Build history of the part. All positions in model axes, mm. Face numbers are marked on the shaded views. A direction names the side the tool comes from. Give positions to 0.01 mm unless a question says otherwise; leave off trailing zeros. Loops run counter-clockwise (first coordinate to the right, second up) from the corner with the lowest first, then second, coordinate; pieces in that order, holes last.
1) Wall check: line 1 (Y direction, x = 33.25, z = 46); line 2 (Y direction, x = 32.25, z = 42); line 3 (Y direction, x = 42.25, z = 41). Give the ranges that are in metal, low to high.
2) Band-saw the part on B-B on x = 37. State how many separate pieces and enclosed holes the cut face has, then the cut area to 3 significant figures.
3) Flat gauge pins, fed straight in: P1, Ø4.5, axis at y = 71.37, z = 65, coming from the -X side; P2, Ø5, axis at x = 43, z = 27.5, coming from the -Y side. Where does each tip first touch, or does it go through?
4) Two-plate mould, pull along Z, no slides. Class the marked faces 1, 2, 3 and 4: +Z half, -Z half, draft (parallel to the pull), parting line (faces both ways), or undercut.
5) Band-saw the part on A-A on z = 27. List the corners of the cut face in (x, y).
6) 3-axis set-ups, long thin cutter, end or side, ignore diameter. For the marked faces 5 and 6: which of +Z, -Z, +X, -X, +Y, -Y reach the whole face in a straight line?
```python
from build123d import *

# Parameters (mm, degrees)
ESQUISSE1_W                   = 15
ESQUISSE1_H                   = 90
BOSS_EXTRU_1_DEPTH            = 80
ESQUISSE2_W                   = 47.5
ESQUISSE2_H                   = 41
ENL_V_MAT_EXTRU_1_DEPTH       = 115.38963181
CONG_1_R                      = 8
ESQUISSE3_W                   = 80
ESQUISSE3_H                   = 85
BOSS_EXTRU_2_DEPTH            = 15
TROU_TARAUD_M5X0_81_D         = 4.2
TROU_TARAUD_PROFOND_M6X1_01_D = 5
R_P_TITION_LIN_AIRE1_COUNT    = 2
R_P_TITION_LIN_AIRE1_PITCH    = 25


with BuildPart() as part:
    # Esquisse1 → Boss.-Extru.1 (new body)
    with BuildSketch(Plane.XY):
        with Locations((37.299465669, 35.374049703)):
            Rectangle(ESQUISSE1_W, ESQUISSE1_H)
    extrude(amount=BOSS_EXTRU_1_DEPTH)

    # Esquisse2 → Enlèv. mat.-Extru.1 (cut, through all)
    with BuildSketch(Plane(origin=(44.799465669, 0, 0), x_dir=(0, 0, -1), z_dir=(1, 0, 0))):
        with Locations((-40, 10.874049703)):
            Rectangle(ESQUISSE2_W, ESQUISSE2_H)
    extrude(amount=-ENL_V_MAT_EXTRU_1_DEPTH, mode=Mode.SUBTRACT)

    # Congé1
    cong_1_edges = [part.edges().sort_by_distance(p)[0] for p in [
        (37.299465669, -9.625950297, 63.75),
        (37.299465669, 31.374049703, 63.75),
        (37.299465669, 31.374049703, 16.25),
        (37.299465669, -9.625950297, 16.25),
    ]]
    fillet(cong_1_edges, radius=CONG_1_R)

    # Esquisse3 → Boss.-Extru.2 (add)
    with BuildSketch(Plane.ZY.offset(-29.799465669)):
        with Locations((40, 122.874049703)):
            Rectangle(ESQUISSE3_W, ESQUISSE3_H)
        with BuildLine():
            Line((12.5, 93.124049703), (67.5, 93.124049703))
            ThreePointArc((67.5, 93.124049703), (70.25, 90.374049703), (67.5, 87.624049703))
            Line((67.5, 87.624049703), (12.5, 87.624049703))
            ThreePointArc((12.5, 87.624049703), (9.75, 90.374049703), (12.5, 93.124049703))
        make_face(mode=Mode.SUBTRACT)
        with BuildLine():
            Line((12.5, 153.124049703), (67.5, 153.124049703))
            ThreePointArc((67.5, 153.124049703), (70.25, 150.374049703), (67.5, 147.624049703))
            Line((67.5, 147.624049703), (12.5, 147.624049703))
            ThreePointArc((12.5, 147.624049703), (9.75, 150.374049703), (12.5, 153.124049703))
        make_face(mode=Mode.SUBTRACT)
    extrude(amount=-BOSS_EXTRU_2_DEPTH)

    # Trou taraudé M5x0.81 (through all)
    with Locations(Plane(origin=(37.299465669, -2.625950297, 80), x_dir=(1, 0, 0), z_dir=(0, 0, 1))):
        with Locations((0, 0), (0, 30)):
            trou_taraud_m5x0_81 = Hole(TROU_TARAUD_M5X0_81_D / 2)

    # Symétrie1: Trou taraudé M5x0.81 across plane
    add(trou_taraud_m5x0_81.mirror(Plane.XY.offset(40)), mode=Mode.SUBTRACT)

    # Trou taraudé profond M6x1.01 (through all)
    with Locations(Plane(origin=(29.799465669, 46.374049703, 15), x_dir=(0, -1, 0), z_dir=(-1, 0, 0))):
        with Locations((0, 0), (0, 25), (0, 50)):
            trou_taraud_profond_m6x1_01 = Hole(TROU_TARAUD_PROFOND_M6X1_01_D / 2)

    # Répétition linéaire1: Trou taraudé profond M6x1.01 ×2
    with Locations(*[(0, i * R_P_TITION_LIN_AIRE1_PITCH, 0) for i in range(1, R_P_TITION_LIN_AIRE1_COUNT)]):
        add(trou_taraud_profond_m6x1_01, mode=Mode.SUBTRACT)


solid = part.part
```
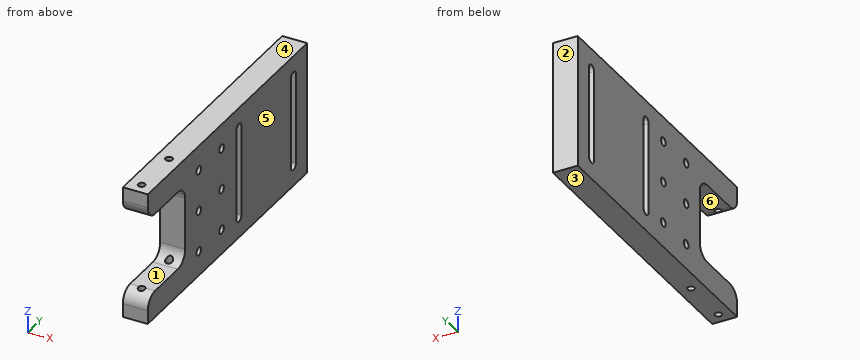
Findings below:
1. line 1: y = 31.37 to 87.62, 93.12 to 147.62, 153.12 to 165.37
1. line 2: y = 31.37 to 44.87, 47.87 to 69.87, 72.87 to 87.62, 93.12 to 147.62, 153.12 to 165.37
1. line 3: y = 31.37 to 44.08, 48.67 to 69.08, 73.67 to 87.62, 93.12 to 147.62, 153.12 to 165.37
2. separate pieces: 5
2. enclosed holes: 8
2. area: 11,000 mm2
3. P1: passes through
3. P2: stops at y = 31.37
4. face 1: undercut
4. face 2: draft
4. face 3: -Z half
4. face 4: +Z half
5. outline: (29.8, 31.37) - (44.8, 31.37) - (44.8, 87.62) - (29.8, 87.62) - close; (29.8, 93.12) - (44.8, 93.12) - (44.8, 147.62) - (29.8, 147.62) - close; (29.8, 153.12) - (44.8, 153.12) - (44.8, 165.37) - (29.8, 165.37) - close
6. face 5: +Z, -Z, +X, +Y, -Y
6. face 6: +X, -X, -Y
